Source: CAD feature listing. Evaluate the final solid. Frame: model axes, mm. Coordinates: 2 decimals unless noted, no trailing zeros. Order: outer loops, then holes, each group sorted by start corner. A loop starts at its lowest first (then second) coordinate and runs counter-clockwise, first axis right, second up.
Item 1: Section D-D on z = -3.25. Return the cut outline in (x, y), then the cut area to 3 significant figures.
Item 2: Section A-A on x = 28. Return the cut outline in (y, z).
Item 3: Section B-B on y = -60.5. Return the cut outline in (x, z), then the cut area to 4 significant figures.
Item 4: Section C-C on x = -28. Return the cut outline in (y, z), then the cut area to 3 significant figures.
Item 5: Ray query, line 1 (Y direction, x = 28, z = -2.9); line 2 (Y direction, x = -27.5, z = -1.95); line 3 (Y direction, x = -28, z = -2.55). Return the intervals inside material, ascending.
from build123d import *

# Parameters (mm, degrees)
SKETCH_1_R             = 5.25
SM_BASE_FLANGE_1_DEPTH = 6


# Sheet-metal steps are written as plain solids
with BuildPart() as part:
    # Sketch 1 → Базовая кромка1 (new body)
    with BuildSketch(Plane.XY):
        Polygon((-41, -102.5), (-56, -87.5), (-56, -18.731551379), (-15, 3.62230522), (-15, 35), (0, 50), (41, 50), (56, 35), (56, -87.5), (41, -102.5), align=None)
        with Locations((-28, -62.5)):
            Circle(SKETCH_1_R, mode=Mode.SUBTRACT)
        with Locations((28, -62.5)):
            Circle(SKETCH_1_R, mode=Mode.SUBTRACT)
        with Locations((28, -31.72618932)):
            Circle(SKETCH_1_R, mode=Mode.SUBTRACT)
    extrude(amount=-SM_BASE_FLANGE_1_DEPTH)


solid = part.part
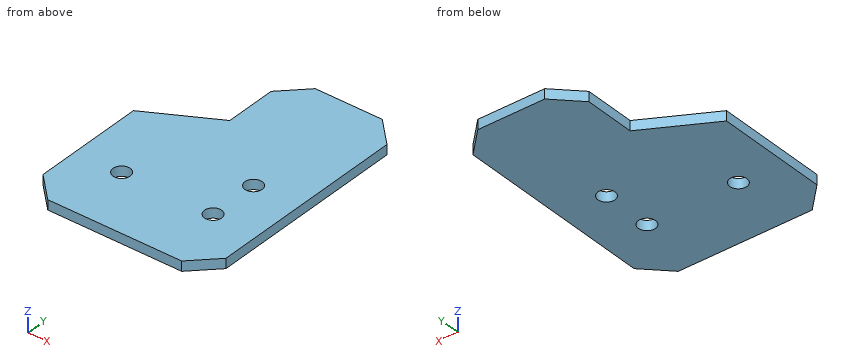
Answer list:
1. outline: (-56, -87.5) - (-41, -102.5) - (41, -102.5) - (56, -87.5) - (56, 35) - (41, 50) - (0, 50) - (-15, 35) - (-15, 3.62) - (-56, -18.73) - close; hole circle Ø10.5 at (-28, -62.5); hole circle Ø10.5 at (28, -62.5); hole circle Ø10.5 at (28, -31.73)
1. area: 14,000 mm2
2. outline: (-102.5, -6) - (-67.75, -6) - (-67.75, 0) - (-102.5, 0) - close; (-57.25, -6) - (-36.98, -6) - (-36.98, 0) - (-57.25, 0) - close; (-26.48, -6) - (50, -6) - (50, 0) - (-26.48, 0) - close
3. outline: (-56, -6) - (-32.85, -6) - (-32.85, 0) - (-56, 0) - close; (-23.15, -6) - (23.15, -6) - (23.15, 0) - (-23.15, 0) - close; (32.85, -6) - (56, -6) - (56, 0) - (32.85, 0) - close
3. area: 555.5 mm2
4. outline: (-102.5, -6) - (-67.75, -6) - (-67.75, 0) - (-102.5, 0) - close; (-57.25, -6) - (-3.47, -6) - (-3.47, 0) - (-57.25, 0) - close
4. area: 531 mm2
5. line 1: y = -102.5 to -67.75, -57.25 to -36.98, -26.48 to 50
5. line 2: y = -102.5 to -67.73, -57.27 to -3.19
5. line 3: y = -102.5 to -67.75, -57.25 to -3.47
